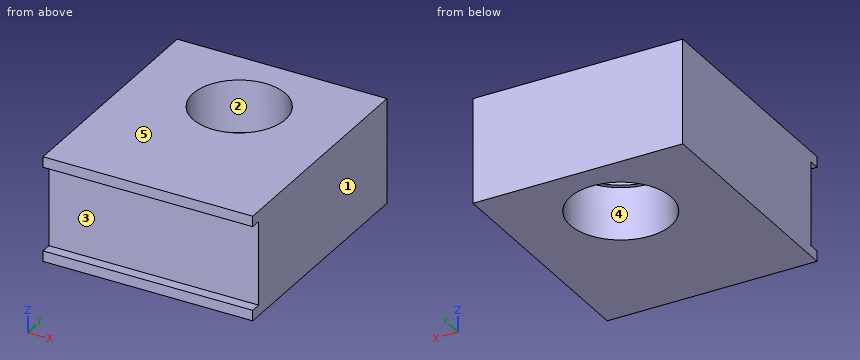
from build123d import *

# Parameters (mm, degrees)
SKETCH1_W           = 32
SKETCH1_H           = 16
BOSS_EXTRUDE1_DEPTH = 36
SKETCH2_W           = 32
SKETCH2_H           = 12.8
CUT_EXTRUDE1_DEPTH  = 1.6
SKETCH3_R           = 7.05
CUT_EXTRUDE2_DEPTH  = 44.036739415
SKETCH4_R           = 7.7
CUT_EXTRUDE3_DEPTH  = 8


with BuildPart() as part:
    # Sketch1 → Boss-Extrude1 (new body)
    with BuildSketch(Plane(origin=(0, 0, 0), x_dir=(1, 0, 0), z_dir=(0, 1, 0))):
        with Locations((1.325153374, -1.104294479)):
            Rectangle(SKETCH1_W, SKETCH1_H)
    extrude(amount=BOSS_EXTRUDE1_DEPTH)

    # Sketch2 → Cut-Extrude1 (cut)
    with BuildSketch(Plane(origin=(0, 0, 0), x_dir=(-1, 0, 0), z_dir=(0, -1, 0))):
        with Locations((-1.325153374, -1.104294479)):
            Rectangle(SKETCH2_W, SKETCH2_H)
    extrude(amount=-CUT_EXTRUDE1_DEPTH, mode=Mode.SUBTRACT)

    # Sketch3 → Cut-Extrude2 (cut, through all)
    with BuildSketch(Plane(origin=(0, 0, -6.895705521), x_dir=(-1, 0, 0), z_dir=(0, 0, -1))):
        with Locations((-1.325153374, 24.5)):
            Circle(SKETCH3_R)
    extrude(amount=-CUT_EXTRUDE2_DEPTH, mode=Mode.SUBTRACT)

    # Sketch4 → Cut-Extrude3 (cut)
    with BuildSketch(Plane(origin=(0, 0, -6.895705521), x_dir=(-1, 0, 0), z_dir=(0, 0, -1))):
        with Locations((-1.325153374, 24.5)):
            Circle(SKETCH4_R)
    extrude(amount=-CUT_EXTRUDE3_DEPTH, mode=Mode.SUBTRACT)


solid = part.part
The model under review builds one solid part; all positions refer to its coordinate system, in mm. Face numbers are marked on the shaded views. A direction names the side the tool comes from. Round coordinates to 2 decimals unless told otherwise and drop trailing zeros. Write each loop counter-clockwise with the first axis right and the second up, starting at its lowest first coordinate (ties: lowest second). Pieces come first, ordered by that corner, then holes. Notation, with made-up numbers: M -33.75,34 L -11.75,34 A4 cw -11.75,38 Z; hole C 88,-13.75 d7. An arc over 180 degrees is marked long. Use a Markdown table: item, result. Add a question column.
Q1. Insertion check: pin 1 (5 mm diameter, centred on x = 1, z = 1, fed in from -Y). The pin has a flat end and moves straight along its axis. Give the tip position at first contact, or say it passes through.
Q2. To check wall thickness, follow line 1 (Y direction, x = 2, z = -2); line 2 (X direction, y = 25.5, z = -3); line 3 (Z direction, x = -2, y = 18). State the ranges of each line that lie inside material, in increasing order.
Q3. We need section D-D, the plane x = -10. State the section outline as (y, z) points.
Q4. We need section A-A, the plane z = 1.75. State the section outline as (x, y) points, plus the area to 3 significant figures.
Q5. We need section C-C, the plane x = 7. State the section outline as (y, z) points.
Q6. Machinability: for the marked faces 4 and 5, which of the approach directions +Z, -Z, +X, -X, +Y, -Y give a long, thin tool a straight path to every point of the face, cutting with its end or side? Answer none if there is none.
Q7. The part is to be moulded in two halves that separate along Y. For the marked faces 1, 2 and 3, say which applies: pulls with the +Y half, pulls with the -Y half, needs draft (parallel to the pull), parting line crosses it, or undercut.
Q8. We need section B-B, the plane y = 24.5. State the section outline as (x, z) points.
Findings below:
| question | item | result |
|---|---|---|
| 1 | pin 1 | stops at y = 1.6 |
| 2 | line 1 | y = 1.6 to 16.83, 32.17 to 36 |
| 2 | line 2 | x = -14.67 to -6.31, 8.96 to 17.33 |
| 2 | line 3 | z = 1.1 to 9.1 |
| 3 | outline | M 0,-6.9 L 36,-6.9 L 36,9.1 L 0,9.1 L 0,7.5 L 1.6,7.5 L 1.6,-5.3 L 0,-5.3 Z |
| 4 | outline | M -14.67,1.6 L 17.33,1.6 L 17.33,36 L -14.67,36 Z; hole C 1.33,24.5 d14.1 |
| 4 | area | 945 mm² |
| 5 | outline | M 0,-6.9 L 19.3,-6.9 L 19.3,1.1 L 20.32,1.1 L 20.32,9.1 L 0,9.1 L 0,7.5 L 1.6,7.5 L 1.6,-5.3 L 0,-5.3 Z; M 28.68,1.1 L 29.7,1.1 L 29.7,-6.9 L 36,-6.9 L 36,9.1 L 28.68,9.1 Z |
| 6 | face 4 | -Z |
| 6 | face 5 | +Z, +X, -X, +Y, -Y |
| 7 | face 1 | needs draft |
| 7 | face 2 | undercut |
| 7 | face 3 | pulls with the -Y half |
| 8 | outline | M -14.67,-6.9 L -6.37,-6.9 L -6.37,1.1 L -5.72,1.1 L -5.72,9.1 L -14.67,9.1 Z; M 8.38,1.1 L 9.03,1.1 L 9.03,-6.9 L 17.33,-6.9 L 17.33,9.1 L 8.38,9.1 Z |
